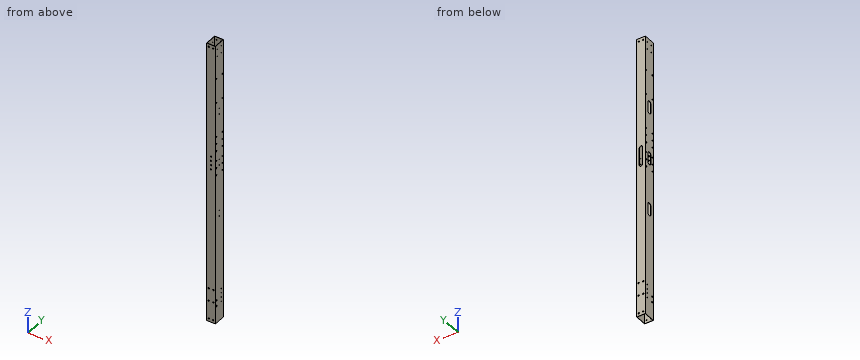
from build123d import *

# Parameters (mm, degrees)
SKETCH_1_W           = 30
SKETCH_1_H           = 40
SKETCH_1_W_2         = 28
SKETCH_1_H_2         = 38
EXTRUDE_1_DEPTH      = 940
SKETCH_5_R           = 2.5
CUT_EXTRUDE_3_DEPTH  = 941.97024395
CUT_EXTRUDE_4_DEPTH  = 1
SKETCH_7_R           = 1.5
CUT_EXTRUDE_5_DEPTH  = 1
SKETCH_17_W          = 30
SKETCH_17_H          = 40
SKETCH_17_W_2        = 28
SKETCH_17_H_2        = 38
EXTRUDE_2_DEPTH      = 20
SKETCH_18_W          = 30
SKETCH_18_H          = 40
SKETCH_18_W_2        = 28
SKETCH_18_H_2        = 38
EXTRUDE_3_DEPTH      = 20
SKETCH_19_R          = 2.1
CUT_EXTRUDE_16_DEPTH = 961.950050731
SKETCH_20_R          = 1.6
CUT_EXTRUDE_17_DEPTH = 961.67684473
SKETCH_21_R          = 2.5
SKETCH_21_R_2        = 1.6
CUT_EXTRUDE_18_DEPTH = 961.67684473
SKETCH_23_R          = 2.5
CUT_EXTRUDE_19_DEPTH = 961.950050731
SKETCH_24_R          = 4.5
CUT_EXTRUDE_20_DEPTH = 10
SKETCH_25_W          = 114.67616049
SKETCH_25_H          = 1154.562704257
CUT_EXTRUDE_21_DEPTH = 968.690549711
SKETCH_26_R          = 2
CUT_EXTRUDE_22_DEPTH = 961.67684473
CUT_EXTRUDE_23_DEPTH = 10


with BuildPart() as part:
    # Sketch 1 → Extrude 1 (new body)
    with BuildSketch(Plane.XY):
        Rectangle(SKETCH_1_W, SKETCH_1_H)
        Rectangle(SKETCH_1_W_2, SKETCH_1_H_2, mode=Mode.SUBTRACT)
    extrude(amount=EXTRUDE_1_DEPTH)

    # Sketch 5 → Cut-Extrude 3 (cut, through all)
    with BuildSketch(Plane.XZ.offset(20)):
        with Locations(Location((-8, 53, 0), (0, 0, 270))):
            Circle(SKETCH_5_R)
        with Locations(Location((8, 53, 0), (0, 0, 270))):
            Circle(SKETCH_5_R)
        with Locations(Location((-8, 97, 0), (0, 0, 270))):
            Circle(SKETCH_5_R)
        with Locations(Location((8, 97, 0), (0, 0, 270))):
            Circle(SKETCH_5_R)
    extrude(amount=-CUT_EXTRUDE_3_DEPTH, mode=Mode.SUBTRACT)

    # Sketch 6 → Cut-Extrude 4 (cut)
    with BuildSketch(Plane(origin=(15, 0, 0), x_dir=(0, 0, -1), z_dir=(1, 0, 0))):
        with BuildLine():
            Line((-345, -7.5), (-375, -7.5))
            ThreePointArc((-375, -7.5), (-382.5, 0), (-375, 7.5))
            Line((-375, 7.5), (-345, 7.5))
            ThreePointArc((-345, 7.5), (-337.5, 0), (-345, -7.5))
        make_face()
        with BuildLine():
            Line((-525, -7.5), (-555, -7.5))
            ThreePointArc((-555, -7.5), (-562.5, 0), (-555, 7.5))
            Line((-555, 7.5), (-525, 7.5))
            ThreePointArc((-525, 7.5), (-517.5, 0), (-525, -7.5))
        make_face()
        with BuildLine():
            Line((-705, -7.5), (-735, -7.5))
            ThreePointArc((-735, -7.5), (-742.5, 0), (-735, 7.5))
            Line((-735, 7.5), (-705, 7.5))
            ThreePointArc((-705, 7.5), (-697.5, 0), (-705, -7.5))
        make_face()
    extrude(amount=-CUT_EXTRUDE_4_DEPTH, mode=Mode.SUBTRACT)

    # Sketch 7 → Cut-Extrude 5 (cut)
    with BuildSketch(Plane.ZY.offset(15)):
        with Locations((350, 0)):
            Circle(SKETCH_7_R)
        with Locations((370, 0)):
            Circle(SKETCH_7_R)
        with Locations((530, 0)):
            Circle(SKETCH_7_R)
        with Locations((550, 0)):
            Circle(SKETCH_7_R)
        with Locations((710, 0)):
            Circle(SKETCH_7_R)
        with Locations((730, 0)):
            Circle(SKETCH_7_R)
    extrude(amount=-CUT_EXTRUDE_5_DEPTH, mode=Mode.SUBTRACT)

    # Sketch 17 → Extrude 2 (add)
    with BuildSketch(Plane.XY.offset(940)):
        Rectangle(SKETCH_17_W, SKETCH_17_H)
        Rectangle(SKETCH_17_W_2, SKETCH_17_H_2, mode=Mode.SUBTRACT)
    extrude(amount=EXTRUDE_2_DEPTH)

    # Sketch 18 → Extrude 3 (add)
    with BuildSketch(Plane(origin=(0, 0, 0), x_dir=(-1, 0, 0), z_dir=(0, 0, -1))):
        Rectangle(SKETCH_18_W, SKETCH_18_H)
        Rectangle(SKETCH_18_W_2, SKETCH_18_H_2, mode=Mode.SUBTRACT)
    extrude(amount=EXTRUDE_3_DEPTH)

    # Sketch 19 → Cut-Extrude 16 (cut, through all)
    with BuildSketch(Plane(origin=(0, 20, 0), x_dir=(1, 0, 0), z_dir=(0, 1, 0))):
        with Locations(Location((-7.5, -950, 0), (0, 0, 270))):
            Circle(SKETCH_19_R)
        with Locations(Location((7.5, -950, 0), (0, 0, 270))):
            Circle(SKETCH_19_R)
        with Locations(Location((-7.5, 10, 0), (0, 0, 270))):
            Circle(SKETCH_19_R)
        with Locations(Location((7.5, 10, 0), (0, 0, 270))):
            Circle(SKETCH_19_R)
    extrude(amount=-CUT_EXTRUDE_16_DEPTH, mode=Mode.SUBTRACT)

    # Sketch 20 → Cut-Extrude 17 (cut, through all)
    with BuildSketch(Plane(origin=(15, 0, 0), x_dir=(0, 0, -1), z_dir=(1, 0, 0))):
        with Locations((-945, 10)):
            Circle(SKETCH_20_R)
        with Locations((-920, 10)):
            Circle(SKETCH_20_R)
        with Locations((-920, -10)):
            Circle(SKETCH_20_R)
        with Locations((-945, -10)):
            Circle(SKETCH_20_R)
    extrude(amount=-CUT_EXTRUDE_17_DEPTH, mode=Mode.SUBTRACT)

    # Sketch 21 → Cut-Extrude 18 (cut, through all)
    with BuildSketch(Plane(origin=(15, 0, 0), x_dir=(0, 0, -1), z_dir=(1, 0, 0))):
        with Locations((-40, -14)):
            Circle(SKETCH_21_R)
        with Locations((-60, -14)):
            Circle(SKETCH_21_R)
        with Locations((-42.5, 10)):
            Circle(SKETCH_21_R_2)
        with Locations((-57.5, 10)):
            Circle(SKETCH_21_R_2)
        with Locations((-72.5, 10)):
            Circle(SKETCH_21_R_2)
        with Locations((-87.5, 10)):
            Circle(SKETCH_21_R_2)
    extrude(amount=-CUT_EXTRUDE_18_DEPTH, mode=Mode.SUBTRACT)

    # Sketch 23 → Cut-Extrude 19 (cut, through all)
    with BuildSketch(Plane(origin=(0, 20, 0), x_dir=(1, 0, 0), z_dir=(0, 1, 0))):
        with Locations(Location((0, -520, 0), (0, 0, 270))):
            Circle(SKETCH_23_R)
        with Locations(Location((0, -535, 0), (0, 0, 270))):
            Circle(SKETCH_23_R)
        with Locations(Location((0, -550, 0), (0, 0, 270))):
            Circle(SKETCH_23_R)
        with Locations(Location((0, -565, 0), (0, 0, 270))):
            Circle(SKETCH_23_R)
    extrude(amount=-CUT_EXTRUDE_19_DEPTH, mode=Mode.SUBTRACT)

    # Sketch 24 → Cut-Extrude 20 (cut)
    with BuildSketch(Plane(origin=(0, 20, 0), x_dir=(1, 0, 0), z_dir=(0, 1, 0))):
        with Locations(Location((0, -520, 0), (0, 0, 270))):
            Circle(SKETCH_24_R)
        with Locations(Location((0, -535, 0), (0, 0, 270))):
            Circle(SKETCH_24_R)
        with Locations(Location((0, -550, 0), (0, 0, 270))):
            Circle(SKETCH_24_R)
        with Locations(Location((0, -565, 0), (0, 0, 270))):
            Circle(SKETCH_24_R)
    extrude(amount=-CUT_EXTRUDE_20_DEPTH, mode=Mode.SUBTRACT)


with BuildPart() as body_2:
    # Mirror 2: mirrored copy
    add(part.part.mirror(Plane(origin=(-50, 0, 0), x_dir=(0, 0, 1), z_dir=(1, 0, 0))))

    # Sketch 26 → Cut-Extrude 22 (cut, through all)
    with BuildSketch(Plane.ZY.offset(115)):
        with Locations((612.5, 15)):
            Circle(SKETCH_26_R)
        with Locations((612.5, -15)):
            Circle(SKETCH_26_R)
        with Locations((527.5, 15)):
            Circle(SKETCH_26_R)
        with Locations((527.5, -15)):
            Circle(SKETCH_26_R)
        with Locations((842.5, 15)):
            Circle(SKETCH_26_R)
        with Locations((842.5, -15)):
            Circle(SKETCH_26_R)
        with Locations((757.5, 15)):
            Circle(SKETCH_26_R)
        with Locations((757.5, -15)):
            Circle(SKETCH_26_R)
        with Locations((637.5, 15)):
            Circle(SKETCH_26_R)
        with Locations((637.5, -15)):
            Circle(SKETCH_26_R)
        with Locations((552.5, -15)):
            Circle(SKETCH_26_R)
        with Locations((552.5, 15)):
            Circle(SKETCH_26_R)
        with Locations((502.5, 15)):
            Circle(SKETCH_26_R)
        with Locations((502.5, -15)):
            Circle(SKETCH_26_R)
        with Locations((587.5, -15)):
            Circle(SKETCH_26_R)
        with Locations((587.5, 15)):
            Circle(SKETCH_26_R)
    extrude(amount=-CUT_EXTRUDE_22_DEPTH, mode=Mode.SUBTRACT)

    # Sketch 27 → Cut-Extrude 23 (cut)
    with BuildSketch(Plane(origin=(0, 20, 0), x_dir=(1, 0, 0), z_dir=(0, 1, 0))):
        with BuildLine():
            Line((-94, -512.5), (-94, -572.5))
            ThreePointArc((-94, -572.5), (-100, -578.5), (-106, -572.5))
            Line((-106, -572.5), (-106, -512.5))
            ThreePointArc((-106, -512.5), (-100, -506.5), (-94, -512.5))
        make_face()
    extrude(amount=-CUT_EXTRUDE_23_DEPTH, mode=Mode.SUBTRACT)


with BuildPart() as part_1:
    add(part.part)

    # Sketch 25 → Cut-Extrude 21 (cut, through all)
    with BuildSketch(Plane(origin=(0, 20, 0), x_dir=(1, 0, 0), z_dir=(0, 1, 0))):
        with Locations((7.338080245, -506.215166959)):
            Rectangle(SKETCH_25_W, SKETCH_25_H)
    extrude(amount=-CUT_EXTRUDE_21_DEPTH, mode=Mode.SUBTRACT)


solid = body_2.part
Work out the finished part from the listing and answer in its coordinate system (mm). Give positions to 0.01 mm unless a question says otherwise; leave off trailing zeros. Order: outer loops, then holes, each group sorted by start corner. A loop starts at its lowest first (then second) coordinate and runs counter-clockwise, first axis right, second up. Notation, with made-up numbers: (-16, -3.5) - (32, -3.5) arc R26 cw to (32, 19.5) - close; hole circle Ø9 at (25, 86.25). An arc over 180 degrees is marked (long way). Answer as CSV lines item,"result". Start each with the question number.
Q1. The part is cut by section A-A (z = 441.5). Write down the section's boundary in (x, y), then the cut area to 3 significant figures.
Q2. Find the intervals of material crossed by L1, parallel to Y at x = -99, z = 496; L2, parallel to X at y = -11, z = 379.5; L3, parallel to Z at x = -92.5, y = 19.6, in increasing order. Write a range as [from, to].
Q3. Given pin 1 Ø1.9 at (y, z) = (-10, 920) entering from +X, flat-ended and moving along its own axis, determine where the tip first touches the part or whether it passes through.
Check result:
1,outline,"(-115, -20) - (-85, -20) - (-85, 20) - (-115, 20) - close; hole (-114, -19) - (-86, -19) - (-86, 19) - (-114, 19) - close"
1,area,"136 mm²"
2,L1,"y = [-20, -19], [19, 20]"
2,L2,"x = [-115, -114], [-86, -85]"
2,L3,"z = [-20, -12.1], [-7.9, 50.55], [55.45, 94.55], [99.45, 947.9], [952.1, 960]"
3,pin 1,"passes through"
